```python
from build123d import *

# Parameters (mm, degrees)
BOSS_EXTRUDE1_DEPTH   = 10
M4_CLEARANCE_HOLE1_D  = 4.5
F_2_0MM_DOWEL_HOLE1_D = 2
FILLET1_R             = 10
FILLET2_R             = 2.5


with BuildPart() as part:
    # Sketch1 → Boss-Extrude1 (new body)
    with BuildSketch(Plane(origin=(0, 0, 0), x_dir=(0, 0, -1), z_dir=(1, 0, 0))):
        with BuildLine():
            Line((-27.833971588, 109.065439697), (-27.833971588, 84.065439697))
            Line((-27.833971588, 84.065439697), (33.366028214, 84.065439697))
            Line((33.366028214, 84.065439697), (33.366028214, 80.065439697))
            Line((33.366028214, 80.065439697), (58.366028214, 80.065439697))
            Line((58.366028214, 80.065439697), (58.366028214, 160.265439697))
            Line((58.366028214, 160.265439697), (54.366028214, 160.265439697))
            Line((54.366028214, 160.265439697), (-27.833971588, 160.265439697))
            ThreePointArc((-27.833971588, 160.265439697), (-167.840009366, 102.273040036), (-225.832409027, -37.732997742))
            Line((-225.832409027, -37.732997742), (-225.832409027, -119.932997544))
            Line((-225.832409027, -119.932997544), (-84.083971786, -119.932997544))
            Line((-84.083971786, -119.932997544), (-84.083971786, -58.732997742))
            Line((-84.083971786, -58.732997742), (-80.083971786, -58.732997742))
            Line((-80.083971786, -58.732997742), (-80.083971786, -33.732997742))
            Line((-80.083971786, -33.732997742), (-174.577902415, -33.732997742))
            ThreePointArc((-174.577902415, -33.732997742), (-130.212161367, 67.473881749), (-27.833971588, 109.065439697))
        make_face()
    extrude(amount=BOSS_EXTRUDE1_DEPTH)

    # M4 Clearance Hole1 (through all)
    with Locations(Plane(origin=(10, 0, 0), x_dir=(0, 0, -1), z_dir=(1, 0, 0))):
        with Locations((-156.283971786, -57.932997742), (-88.283971786, -57.932997742), (34.166028214, 156.265439697), (34.166028214, 88.265439697)):
            Hole(M4_CLEARANCE_HOLE1_D / 2)

    # Ø2.0mm Dowel Hole1 (through all)
    with Locations(Plane(origin=(10, 0, 0), x_dir=(0, 0, -1), z_dir=(1, 0, 0))):
        with Locations((44.366028214, 83.065439697), (55.366028214, 94.065439697), (55.366028214, 150.265439697), (-150.283971786, -36.732997742), (-93.083971786, -36.732997742), (-83.083971786, -46.732997742)):
            Hole(F_2_0MM_DOWEL_HOLE1_D / 2)

    # Fillet1
    # the kernel refuses this fillet: 10 mm, written as the material it adds along each edge
    with BuildSketch(Plane(origin=(0, -58.732997742, 84.083971786), x_dir=(0, 0, -1), z_dir=(1, 0, 0))) as fillet1_piece_1:
        with BuildLine():
            CenterArc((10, -8), FILLET1_R, 126.869897646, 53.130102354)
            Line((0, -8), (0, 0))
            Line((0, 0), (4, 0))
        make_face()
    extrude(amount=10)
    with BuildSketch(Plane(origin=(0, 84.065439697, -33.366028214), x_dir=(0, 0, 1), z_dir=(1, 0, 0))) as fillet1_piece_2:
        with BuildLine():
            CenterArc((8, 10), FILLET1_R, 216.869897646, 53.130102354)
            Line((0, 4), (0, 0))
            Line((0, 0), (8, 0))
        make_face()
    extrude(amount=10)
    with BuildSketch(Plane(origin=(0, -33.732997742, 174.577902415), x_dir=(0, 0.9978956594350473, -0.06484021036896881), z_dir=(1, 0, 0))) as fillet1_piece_3:
        with BuildLine():
            CenterArc((10.670397133, -9.992919204), FILLET1_R, 87.843724259, 95.873954258)
            Line((0.691440539, -10.641321308), (0, 0))
            ThreePointArc((0, 0), (5.523324707, 0.103944977), (11.046649415, 0))
        make_face()
    extrude(amount=10)
    with BuildSketch(Plane(origin=(0, 109.065439697, 27.833971588), x_dir=(0, -1, 0), z_dir=(1, 0, 0))) as fillet1_piece_4:
        with BuildLine():
            CenterArc((10.365990837, -10), FILLET1_R, 90, 94.192074979)
            ThreePointArc((0.392744859, -10.731002502), (0.098219073, -5.369093574), (0, 0))
            Line((0, 0), (10.365990837, 0))
        make_face()
    extrude(amount=10)
    # the kernel refuses this fillet: 10 mm, written as the material it takes off along each edge
    with BuildSketch(Plane(origin=(-25, -119.932997544, 84.083971786), x_dir=(0, 1, 0), z_dir=(1, 0, 0)), Plane(origin=(-25, -33.732997742, 80.083971786), x_dir=(0, 0, 1), z_dir=(1, 0, 0))) as fillet1_2_piece_1:
        with BuildLine():
            CenterArc((FILLET1_R, FILLET1_R), FILLET1_R, 180, 90)
            Line((0, FILLET1_R), (0, 0))
            Line((0, 0), (FILLET1_R, 0))
        make_face()
    extrude(amount=60, mode=Mode.SUBTRACT)
    with BuildSketch(Plane(origin=(-25, 84.065439697, 27.833971588), x_dir=(0, 1, 0), z_dir=(1, 0, 0)), Plane(origin=(-25, 160.265439697, -58.366028214), x_dir=(0, -1, 0), z_dir=(1, 0, 0)), Plane(origin=(-25, 80.065439697, -58.366028214), x_dir=(0, 0, 1), z_dir=(1, 0, 0))) as fillet1_2_piece_2:
        with BuildLine():
            CenterArc((FILLET1_R, -FILLET1_R), FILLET1_R, 90, 90)
            Line((0, -FILLET1_R), (0, 0))
            Line((0, 0), (FILLET1_R, 0))
        make_face()
    extrude(amount=60, mode=Mode.SUBTRACT)

    # Fillet2
    fillet2_edges = [part.edges().sort_by_distance(p)[0] for p in [
        (5, 80.065439697, -33.366028214),
        (5, -58.732997742, 80.083971786),
        (5, -119.932997544, 225.832409027),
    ]]
    fillet(fillet2_edges, radius=FILLET2_R)


solid = part.part
```
Can you work these out from the model? Positions are in its coordinate system, mm. A direction names the side the tool comes from. Give positions to 0.01 mm unless a question says otherwise; leave off trailing zeros. Write each loop counter-clockwise with the first axis right and the second up, starting at its lowest first coordinate (ties: lowest second). Pieces come first, ordered by that corner, then holes. Notation, with made-up numbers: (17, 14.5) -> (47, 14.5) arc R21 cw to (47, 20.5) -> close; hole circle Ø4 at (5, 73). An arc over 180 degrees is marked (long way). Write item = value, one per line.
(1) For faces 4 (the face through (4.93, -36.74, 82.936)), 5 (the face through (4.93, 83.207, -29.419)), 6 (the face through (5, -89, 84.084)), which set-ups out of +Z, -Z, +X, -X, +Y, -Y let a thin tool reach every point of the face, with its end or its side?
Worked out:
face_4 = -Z, +X, -X
face_5 = +X, -X, -Y
face_6 = -Z, +X, -X, -Y
(2) Suppose I cut it at C-C on y = 1.5. Write out the boundary of the cut face in (x, z).
Worked out:
outline = (0, 169.29) -> (10, 169.29) -> (10, 221.91) -> (0, 221.91) -> close
(3) I need wall thicknesses on probe 1 along Y at (x, z) = (4, -44); probe 2 along Z at (x, y) = (2, -60); probe 3 along Z at (x, y) = (9, -49). Which ranges of each line are inside material? Lowest first, please. Write a range as from..to.
Worked out:
probe_1 = 80.07..82.13, 84..160.27
probe_2 = 81.48..87.4, 89.17..155.4, 157.17..225.83
probe_3 = 80.08..225.83
(4) Suppose I cut it at B-B on x = 2.5. Count the separate pieces of the cut face and the enclosed holes in it, then the cut area to 3 significant figures.
Worked out:
separate_pieces = 1
enclosed_holes = 10
area = 32,500 mm^2
(5) Suppose I cut it at D-D on z = 64. Write out the boundary of the cut face in (x, y).
Worked out:
outline = (0, 104.54) -> (10, 104.54) -> (10, 156.93) -> (0, 156.93) -> close
(6) I'm going to push flat-ended pins straight in: P1, Ø2.5, axis at y = -46.73, z = 83.08, coming from the -X side; P2, Ø3, axis at x = 4.5, y = -93.5, coming from the -Z side; P3, Ø3, axis at x = 6.5, z = 118, coming from the +Y side; P4, Ø3, axis at x = 5, y = 5, coming from the -Z side. Where does each tip first touch, or does it pass through?
Worked out:
P1 = 0
P2 = 84.08
P3 = 139.3
P4 = 167.81
(7) Suppose I cut it at A-A on z = 135. Write out the boundary of the cut face in (x, y).
Worked out:
outline = (0, -119.93) -> (10, -119.93) -> (10, -33.73) -> (0, -33.73) -> close; (0, 62.59) -> (10, 62.59) -> (10, 128.76) -> (0, 128.76) -> close
(8) Thinking about a two-plate mould opening in Z: for faces 1 (the face through (4.93, 87.07, 24.98)), 2 (the face through (4.93, -117.08, 87.09)), 3 (the face through (5, 80.065, -41)), which applies, released by +Z, released by -Z, zero draft, split by the parting line, or undercut?
Worked out:
face_1 = undercut
face_2 = released by -Z
face_3 = zero draft
